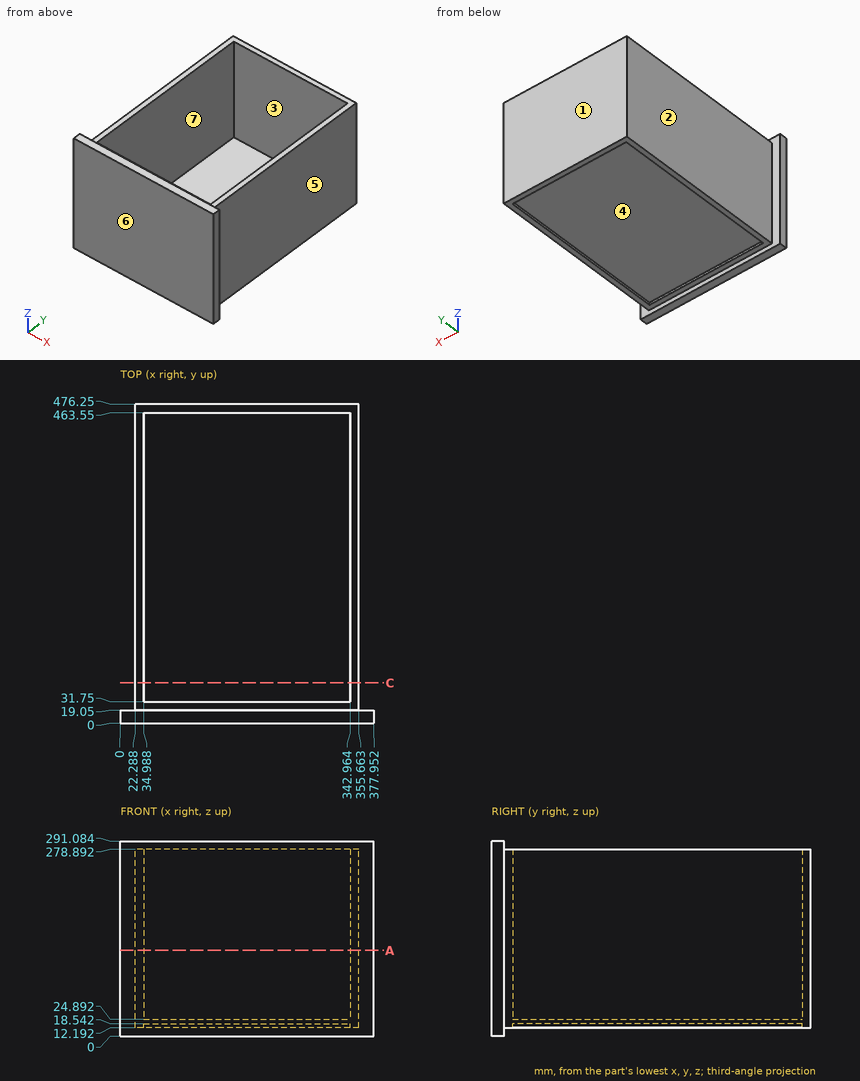
Input: dimensioned drawing with shaded views. Units: mm. Origin: part minimum x, y, z. A direction names the side the tool comes from. Give positions to 0.01 mm unless a question says otherwise; leave off trailing zeros. Order: outer loops, then holes, each group sorted by start corner. A loop starts at its lowest first (then second) coordinate and runs counter-clockwise, first axis right, second up.
(1) Section query C-C (y = 60). Return the cut outline in (x, z).
(2) Contact query for flat-ended pins moving along their axis: P1, Ø5, axis at y = 198.5, z = 14, coming from the +X side; P2, Ø8, axis at x = 325.5, y = 374.5, coming from the +Z side; P3, Ø3, axis at y = 241, z = 16, coming from the -X side. Output: stop coordinate, or through.
(3) Material intervals for line 1 along Y through (x, z) = (53.5, 34); line 2 along X through (y, z) = (457.5, 104); line 3 along Z through (x, y) = (350, 379.5), sorted ascending.
(4) Section query A-A (z = 128). Return the cut outline in (x, y).
(5) Access query for the marked faces 1, 2, 3 and 4. Directions: +Z, -Z, +X, -X, +Y, -Y. A direction counts if a zero-diameter tool reaches every point of the face in a straight line with its end or side. Return the directions, or none.
(6) Pull-direction query (Y, two-part tool) for the marked faces 5, 6 and 7; classes: +Y half, -Y half, draft (parallel to the pull), parting line (faces both ways), or undercut.
Outcome:
1. outline: (22.29, 12.19) - (34.99, 12.19) - (34.99, 18.54) - (342.96, 18.54) - (342.96, 12.19) - (355.66, 12.19) - (355.66, 278.89) - (342.96, 278.89) - (342.96, 24.89) - (34.99, 24.89) - (34.99, 278.89) - (22.29, 278.89) - close
2. P1: stops at x = 355.66
2. P2: stops at z = 24.89
2. P3: stops at x = 22.29
3. line 1: y = 0 to 31.75, 463.55 to 476.25
3. line 2: x = 22.29 to 34.99, 342.96 to 355.66
3. line 3: z = 12.19 to 278.89
4. outline: (0, 0) - (377.95, 0) - (377.95, 19.05) - (355.66, 19.05) - (355.66, 476.25) - (22.29, 476.25) - (22.29, 19.05) - (0, 19.05) - close; hole (34.99, 31.75) - (342.96, 31.75) - (342.96, 463.55) - (34.99, 463.55) - close
5. face 1: +Z, -Z, +X, -X, +Y
5. face 2: +Z, -Z, -X, +Y
5. face 3: +Z
5. face 4: -Z
6. face 5: draft
6. face 6: -Y half
6. face 7: undercut
